The listing builds one solid part. Answer for the finished solid, in the listing's coordinates (mm). A direction names the side the tool comes from. Round coordinates to 2 decimals unless told otherwise and drop trailing zeros. Write each loop counter-clockwise with the first axis right and the second up, starting at its lowest first coordinate (ties: lowest second). Pieces come first, ordered by that corner, then holes.
Autodesk Inventor part; units mm, degrees
ref_plane "YZ Plane" through (0, 0, 0) normal (1, 0, 0) x (0, 1, 0)
ref_plane "XZ Plane" through (0, 0, 0) normal (0, 1, 0) x (-1, 0, 0)
ref_plane "XY Plane" through (0, 0, 0) normal (0, 0, 1) x (1, 0, 0)
sketch "Sketch2" plane through (0, 0, 0) normal (1, 0, 0) x (0, 1, 0)
  line L0 (0, 0) -> (25.4, 0)
  line L1 (25.4, 0) -> (25.4, -114.3)
  line L2 (25.4, -114.3) -> (0, -114.3)
  line L3 (0, -114.3) -> (0, 0)
  dimension "d6" = 25.4
  dimension "d7" = 114.3
extrude "Extrusion2" add sketch "Sketch2" along normal blind 4.7625
sketch "Sketch3" plane through (4.7625, 0, 0) normal (1, 0, 0) x (0, 0, -1)
  line L0 (0, 0) -> (114.3, 0)
  line L1 (0, 0) -> (-14.429, -2.5442)
  line L2 (0, 0) -> (14.6516, 0) construction
  dimension "d10" = 170
ref_plane "Work Plane1" through (4.7625, -2.5442, 14.429) normal (0, 0.9848, 0.1736) x (0, 0.1736, -0.9848)
sketch "Sketch4" plane through (4.7625, -2.5442, 14.429) normal (0, 0.9848, 0.1736) x (0, 0.1736, -0.9848)
  line L0 (127.2151, 4.7625) -> (14.6516, 4.7625)
  line L1 (127.2151, 4.7625) -> (127.2151, 0)
  line L2 (14.6516, 0) -> (127.2151, 0)
  line L3 (14.6516, 4.7625) -> (14.6516, 0)
  arc A0 (11.4766, 4.7625) -> (14.6516, 3.9118) centre (11.4766, -1.5875) ccw
  circle A1 centre (11.4766, -1.5875) radius 3.175
  line L4 (14.6516, 4.7625) -> (11.4766, 4.7625)
  line L5 (14.6516, 4.7625) -> (14.6516, 0)
  dimension "d11" = 12.7
  dimension "d12" = 3.175
  dimension "d13" = 4.7625
  dimension "d15" = 6.35
  dimension "d26" = 1.5875
extrude "Extrusion3" add sketch "Sketch4" along normal blind 6.35 contours L3 L2 A0 L4 | A0 L2 L3
sketch "Sketch5" plane through (0, 25.4, 0) normal (0, 1, 0) x (1, 0, 0)
  line L0 (0, 0) -> (0, 114.3)
  line L1 (0, 0) -> (4.7625, 0)
  line L2 (4.7625, 114.3) -> (4.7625, 0)
  line L3 (0, 114.3) -> (4.7625, 114.3)
  line L4 (0, 114.3) -> (0, 0)
  line L5 (0, 114.3) -> (16.5392, 114.3)
  line L6 (16.5392, 114.3) -> (16.5392, 95.6232)
  line L7 (16.5392, 95.6232) -> (0, 95.6232)
  line L8 (0, 95.6232) -> (0, 114.3)
extrude "Extrusion4" add sketch "Sketch5" against normal blind 3.175 contours L0 L3 L2 L7 | L2 L5 L6 L7
sketch "Sketch6" plane through (4.7625, -2.5442, 14.429) normal (0, 0.9848, 0.1736) x (0, 0.1736, -0.9848)
  line L0 (17.6249, 0) -> (14.6516, 0)
  arc A0 (17.6249, 0) -> (11.4766, 4.7625) centre (11.4766, -1.5875) ccw
  line L1 (14.6516, 3.9118) -> (14.6516, 0)
  circle A1 centre (11.4766, -1.5875) radius 3.175
  line L2 (127.2151, 4.7625) -> (14.6516, 4.7625)
  line L3 (14.6516, -4.7625) -> (8.3016, -4.7625)
  line L4 (8.3016, -4.7625) -> (8.3016, -17.4625)
  line L5 (8.3016, -17.4625) -> (14.6516, -17.4625)
  line L6 (14.6516, -17.4625) -> (14.6516, -4.7625)
  line L7 (14.6516, 4.7625) -> (11.4766, 4.7625)
  line L8 (14.6516, 4.7625) -> (14.6516, 3.9118)
  point P0 (17.3632, 4.7625)
  dimension "d22" = 6.35
  dimension "d23" = 12.7
  dimension "d27" = 0
extrude "Extrusion5" add sketch "Sketch6" along normal blind 6.35 contours L3 L6 L5 L4
equation "\"d26\" = 0.5 * d11 - d13"
properties part number "WheelIntakeMotorMount"
1. Section D-D on z = -43 is taken. Determine the outline of the cut face in (x, y).
Geometry says:
outline: (0, 0) - (4.76, 0) - (4.76, 25.4) - (0, 25.4) - close
2. Section C-C on y = 12.75 is taken. Determine the outline of the cut face in (x, z), plus the area to 3 significant figures.
Geometry says:
outline: (0, -114.3) - (4.76, -114.3) - (4.76, 0) - (0, 0) - close
area: 544 mm2
3. Section A-A on x = 15 is taken. Determine the outline of the cut face in (y, z) (3 decimals), plus the area to 3 significant figures.
Geometry says:
outline: (-1.103, 6.254) - (0, 0) - (6.254, 1.103) - (5.151, 7.356) - close; (22.225, -114.3) - (25.4, -114.3) - (25.4, -95.623) - (22.225, -95.623) - close
area: 99.6 mm2
4. Given pin 1 (1.5 mm diameter, centred on y = 16.5, z = -17.5, fed in from -X); pin 2 (5 mm diameter, centred on x = 14, y = 5, fed in from +Z); pin 3 (6 mm diameter, centred on y = 12, z = -71, fed in from +X); pin 4 (6 mm diameter, centred on x = 7, z = -39, fed in from -Y), each flat-ended and moving along its own axis, determine where each tip first touches the part or whether it passes through.
Geometry says:
pin 1: stops at x = 0
pin 2: stops at z = 7.89
pin 3: stops at x = 4.76
pin 4: stops at y = 0
5. A tool of negligible diameter and unlimited length cuts with its end or side. For faces 4 (the face through (11, 22.225, -105)), 5 (the face through (11, 24, -95.623)), 6 (the face through (17.11, 3.083, 0.544)), from which of +Z, -Z, +X, -X, +Y, -Y can it reach the whole face along a straight path? Write none if from no direction.
Geometry says:
face 4: +Z, -Z, +X, -Y
face 5: +Z, +X, +Y, -Y
face 6: -Z, +X, +Y
6. Straight lines are drawn through the part: line 1 along Z through (x, y) = (2.5, 9.5); line 2 along X through (y, z) = (12, -25.5); line 3 along Y through (x, z) = (7.5, -105) (3 decimals). For each, find the intervals that lie inside material, in ascending order.
Geometry says:
line 1: z = -114.3 to 0
line 2: x = 0 to 4.76
line 3: y = 22.225 to 25.4
7. For a pull along Z with two mould halves and no side action, classify faces 1 (the face through (9.498, 2.46, 4.077)), 2 (the face through (17, 2, 6.8)), 3 (the face through (0, 13, -56)) as released by +Z, released by -Z, zero draft, split by the parting line, or undercut.
Geometry says:
face 1: undercut
face 2: released by +Z
face 3: zero draft
8. Section B-B on z = -103 is taken. Determine the outline of the cut face in (x, y) (1 decimal).
Geometry says:
outline: (0, 0) - (4.8, 0) - (4.8, 22.2) - (16.5, 22.2) - (16.5, 25.4) - (0, 25.4) - close
